from build123d import *

# Parameters (mm, degrees)
ESBO_O1_W                = 289.676219128
ESBO_O1_H                = 190
ESBO_O1_W_2              = 249.676219128
ESBO_O1_H_2              = 150
RESSALTO_EXTRUS_O1_DEPTH = 45
CHANFRO1_SIZE            = 30
CHANFRO2_SIZE            = 10


with BuildPart() as part:
    # Esboço1 → Ressalto-extrusão1 (new body)
    with BuildSketch(Plane.XY):
        Rectangle(ESBO_O1_W, ESBO_O1_H)
        Rectangle(ESBO_O1_W_2, ESBO_O1_H_2, mode=Mode.SUBTRACT)
    extrude(amount=RESSALTO_EXTRUS_O1_DEPTH)

    # Chanfro1
    chanfro1_edges = [part.edges().sort_by_distance(p)[0] for p in [
        (124.838109564, -75, 22.5),
        (124.838109564, 75, 22.5),
        (-124.838109564, 75, 22.5),
        (-124.838109564, -75, 22.5),
        (-144.838109564, 95, 22.5),
        (144.838109564, 95, 22.5),
        (144.838109564, -95, 22.5),
        (-144.838109564, -95, 22.5),
    ]]
    chamfer(chanfro1_edges, length=CHANFRO1_SIZE)

    # Chanfro2
    chanfro2_edges = [part.edges().sort_by_distance(p)[0] for p in [
        (144.838109564, 0, 0),
        (144.838109564, 0, 45),
        (-144.838109564, 0, 0),
        (0, 95, 0),
        (0, -95, 0),
        (-129.838109564, 80, 0),
        (-129.838109564, -80, 0),
        (129.838109564, 80, 0),
        (129.838109564, -80, 0),
        (0, -95, 45),
        (-144.838109564, 0, 45),
        (0, 95, 45),
        (-129.838109564, 80, 45),
        (-129.838109564, -80, 45),
        (129.838109564, 80, 45),
        (129.838109564, -80, 45),
    ]]
    chamfer(chanfro2_edges, length=CHANFRO2_SIZE)


solid = part.part
Geometry check sheet. Reference: the model listing, model coordinates, mm. A direction names the side the tool comes from. Coordinates: 2 decimals unless noted, no trailing zeros. Write each loop counter-clockwise with the first axis right and the second up, starting at its lowest first coordinate (ties: lowest second). Pieces come first, ordered by that corner, then holes. Notation, with made-up numbers: (0.5, 77.5) -> (29.5, 77.5) arc R31 ccw to (29.5, 114.5) -> close; hole circle Ø10 at (73, 62.25). An arc over 180 degrees is marked (long way). One line per question, with ' | ' between items.
1. Cross-section at B-B on x = -75.5. Record the cut outline in (y, z).
Answers:
outline: (-95, 10) -> (-85, 0) -> (-75, 0) -> (-75, 45) -> (-85, 45) -> (-95, 35) -> close; (75, 0) -> (85, 0) -> (95, 10) -> (95, 35) -> (85, 45) -> (75, 45) -> close
2. Cross-section at A-A on y = 19. Record the cut outline in (x, z).
Answers:
outline: (-144.84, 10) -> (-134.84, 0) -> (-124.84, 0) -> (-124.84, 45) -> (-134.84, 45) -> (-144.84, 35) -> close; (124.84, 0) -> (134.84, 0) -> (144.84, 10) -> (144.84, 35) -> (134.84, 45) -> (124.84, 45) -> close
3. Thickness scan on probe 1 along X at (y, z) = (30.5, 29); probe 2 along Y at (x, z) = (-44, 14); probe 3 along X at (y, z) = (46.5, 15). Record the ranges inside material, lowest first. Write a range as from..to.
Answers:
probe 1: x = -144.84..-124.84, 124.84..144.84 | probe 2: y = -95..-75, 75..95 | probe 3: x = -144.84..-123.34, 123.34..144.84
4. Cross-section at C-C on z = 14. Record the cut outline in (x, y), and give its area (3 significant figures).
Answers:
outline: (-144.84, -65) -> (-114.84, -95) -> (114.84, -95) -> (144.84, -65) -> (144.84, 65) -> (114.84, 95) -> (-114.84, 95) -> (-144.84, 65) -> close; hole (-124.84, -45) -> (-94.84, -75) -> (94.84, -75) -> (124.84, -45) -> (124.84, 45) -> (94.84, 75) -> (-94.84, 75) -> (-124.84, 45) -> close | area: 17,600 mm²
5. Cross-section at D-D on z = 38. Record the cut outline in (x, y).
Answers:
outline: (-141.84, -63.76) -> (-113.6, -92) -> (113.6, -92) -> (141.84, -63.76) -> (141.84, 63.76) -> (113.6, 92) -> (-113.6, 92) -> (-141.84, 63.76) -> close; hole (-124.84, -45) -> (-94.84, -75) -> (94.84, -75) -> (124.84, -45) -> (124.84, 45) -> (94.84, 75) -> (-94.84, 75) -> (-124.84, 45) -> close
6. Set-up check for faces 4 (the flat face through (-126.463, -76.205, 40.07)), 5 (the flat face through (124.838, -1, 22)): record each of +Z, -Z, +X, -X, +Y, -Y from which the full face is reachable in a straight line by a thin tool's end or side.
Answers:
face 4: +Z, -X, -Y | face 5: +Z, -Z
7. Draft check along Y on faces 1 (the flat face through (-2, 95, 22)), 2 (the flat face through (109.63, 60.21, 22.18)), 3 (the flat face through (-2, -95, 22)). Enter one of: +Y half, -Y half, draft (parallel to the pull), parting line (faces both ways), or undercut.
Answers:
face 1: +Y half | face 2: undercut | face 3: -Y half
8. Depth check by flat-ended pin: pin 1 Ø5 at (y, z) = (-69, 13.5) entering from +X. Enter the tip coordinate at first touch or a pass-through.
Answers:
pin 1: stops at x = 143.34
